```python
from build123d import *

# Parameters (mm, degrees)
BOSS_EXTRU_1_DEPTH = 6.35
ESQUISSE2_W        = 1.2
ESQUISSE2_H        = 105.4
BOSS_EXTRU_2_DEPTH = 6.35
D_GAGEMENT_1_41_D  = 7.14248


with BuildPart() as part:
    # Esquisse1 → Boss.-Extru.1 (new body)
    with BuildSketch(Plane.XY):
        Polygon((55.8, 113.5), (116.6, 113.5), (116.6, 175.65), (245, 175.65), (245, 113.5), (305.8, 113.5), (305.8, 52.7), (362.1, 52.7), (362.1, -52.7), (305.8, -52.7), (305.8, -113.5), (245, -113.5), (245, -175.65), (116.6, -175.65), (116.6, -113.5), (55.8, -113.5), (55.8, -52.7), (0, -52.7), (0, 52.7), (55.8, 52.7), align=None)
    extrude(amount=BOSS_EXTRU_1_DEPTH)

    # Esquisse2 → Boss.-Extru.2 (add, through all)
    with BuildSketch(Plane.XY.offset(6.35)):
        with Locations((362.7, 0)):
            Rectangle(ESQUISSE2_W, ESQUISSE2_H)
    extrude(amount=-BOSS_EXTRU_2_DEPTH)

    # Dégagement 1/41 (through all)
    with Locations(Plane(origin=(0, 0, 0), x_dir=(-1, 0, 0), z_dir=(0, 0, -1))):
        with Locations((-290.6, 98.3), (-71, 98.3), (-71, -98.3), (-290.6, -98.3)):
            Hole(D_GAGEMENT_1_41_D / 2)


solid = part.part
```
The model under review builds one solid part; all positions refer to its coordinate system, in mm. Coordinates: 2 decimals unless noted, no trailing zeros. Write each loop counter-clockwise with the first axis right and the second up, starting at its lowest first coordinate (ties: lowest second). Pieces come first, ordered by that corner, then holes. Notation, with made-up numbers: (-35, 56) -> (17, 56) arc R15 cw to (17, 69) -> close; hole circle Ø1 at (39, 67.25). An arc over 180 degrees is marked (long way). One line per item, written item: value. Start each with the question number.
Q1. To check wall thickness, follow probe 1 along Y at (x, z) = (290.6, 4.5); probe 2 along X at (y, z) = (-97.5, 1.5); probe 3 along X at (y, z) = (-136.5, 4.25). State the ranges of each line that lie inside material, in increasing order.
Q2. Add section B-B, the plane y = -63. Give the boundary of the cut face in (x, z), then the cut area to 3 significant figures.
Q3. Add section A-A, the plane z = 1. Give the boundary of the cut face in (x, y).
Q4. Clearance check with flat-ended pins moving along their axes: P1, Ø3, axis at y = -147, z = 2.5, coming from the +X side; P2, Ø3, axis at x = 39, z = 3.5, coming from the +Y side; P3, Ø3, axis at y = -153, z = 4, coming from the -X side. State where each tip first meets the part, or that it passes through.
Q5. Add section C-C, the plane x = 60. Give the boundary of the cut face in (y, z), then the cut area to 3 significant figures.
Response:
1. probe 1: -113.5 to -101.87, -94.73 to 94.73, 101.87 to 113.5
1. probe 2: 55.8 to 67.52, 74.48 to 287.12, 294.08 to 305.8
1. probe 3: 116.6 to 245
2. outline: (55.8, 0) -> (305.8, 0) -> (305.8, 6.35) -> (55.8, 6.35) -> close
2. area: 1,590 mm²
3. outline: (0, -52.7) -> (55.8, -52.7) -> (55.8, -113.5) -> (116.6, -113.5) -> (116.6, -175.65) -> (245, -175.65) -> (245, -113.5) -> (305.8, -113.5) -> (305.8, -52.7) -> (363.3, -52.7) -> (363.3, 52.7) -> (305.8, 52.7) -> (305.8, 113.5) -> (245, 113.5) -> (245, 175.65) -> (116.6, 175.65) -> (116.6, 113.5) -> (55.8, 113.5) -> (55.8, 52.7) -> (0, 52.7) -> close; hole circle Ø7.14 at (71, -98.3); hole circle Ø7.14 at (71, 98.3); hole circle Ø7.14 at (290.6, -98.3); hole circle Ø7.14 at (290.6, 98.3)
4. P1: x = 245
4. P2: y = 52.7
4. P3: x = 116.6
5. outline: (-113.5, 0) -> (113.5, 0) -> (113.5, 6.35) -> (-113.5, 6.35) -> close
5. area: 1,440 mm²
